The model under review builds one solid part; all positions refer to its coordinate system, in mm. A direction names the side the tool comes from. Round coordinates to 2 decimals unless told otherwise and drop trailing zeros. Write each loop counter-clockwise with the first axis right and the second up, starting at its lowest first coordinate (ties: lowest second). Pieces come first, ordered by that corner, then holes. Notation, with made-up numbers: (66, -7) - (105, -7) arc R19 cw to (105, 4) - close; hole circle Ø1 at (-2, 79.5). An arc over 180 degrees is marked (long way). Return JSON: item names as keys, results as strings.
from build123d import *
from build123d.topology import SkipClean

# Parameters (mm, degrees)
EXTRUDE_1_DEPTH     = 10
CUT_EXTRUDE_1_DEPTH = 5


with BuildPart() as part:
    # 草圖1 → 填料-伸長1 (new, symmetric)
    with BuildSketch(Plane(origin=(0, 0, 0), x_dir=(1, 0, 0), z_dir=(0, 1, 0))):
        with BuildLine():
            Line((95.00000000000004, 14.999999999999998), (-94.99999999999996, 15))
            ThreePointArc((-94.99999999999996, 14.999999999999998), (-84.39339828220174, 10.606601717798211), (-79.99999999999996, 0))
            ThreePointArc((-79.99999999999996, -3.67e-15), (-84.39339828220174, -10.606601717798204), (-94.99999999999994, -14.999999999999998))
            Line((-94.99999999999994, -14.999999999999961), (95.00000000000006, -14.999999999999998))
            ThreePointArc((95.00000000000004, -14.999999999999998), (80.00000000000004, 1.84e-15), (95.00000000000004, 14.999999999999998))
        make_face()
        with BuildLine():
            ThreePointArc((-79.99999999999996, 0), (-84.39339828220174, 10.606601717798211), (-94.99999999999996, 14.999999999999998))
            Line((-94.99999999999996, 15), (-94.99999999999996, 10.000000000000009))
            ThreePointArc((-95, 10.000000000000009), (-87.9289321881345, 7.071067811865497), (-84.99999999999994, 0))
            ThreePointArc((-84.99999999999994, -2.45e-15), (-87.9289321881345, -7.071067811865502), (-95, -10.000000000000009))
            Line((-94.99999999999994, -10.000000000000007), (-94.99999999999994, -14.999999999999961))
            ThreePointArc((-94.99999999999994, -14.999999999999998), (-84.39339828220174, -10.606601717798204), (-79.99999999999996, -3.67e-15))
        make_face()
        with BuildLine():
            Line((-94.99999999999996, 10.000000000000009), (-94.99999999999996, 15))
            ThreePointArc((-94.99999999999996, 14.999999999999998), (-109.99999999999996, -4.82e-15), (-94.99999999999994, -14.999999999999998))
            Line((-94.99999999999994, -14.999999999999961), (-94.99999999999994, -10.000000000000007))
            ThreePointArc((-95, -10.000000000000009), (-104.99999999999997, 1.22e-15), (-95, 10.000000000000009))
        make_face()
        with BuildLine():
            ThreePointArc((-79.99999999999996, 0), (-84.39339828220174, 10.606601717798211), (-94.99999999999996, 14.999999999999998))
            Line((-94.99999999999996, 15), (-94.99999999999996, 10.000000000000009))
            ThreePointArc((-95, 10.000000000000009), (-87.9289321881345, 7.071067811865497), (-84.99999999999994, 0))
            ThreePointArc((-84.99999999999994, -2.45e-15), (-87.9289321881345, -7.071067811865502), (-95, -10.000000000000009))
            Line((-94.99999999999994, -10.000000000000007), (-94.99999999999994, -14.999999999999961))
            ThreePointArc((-94.99999999999994, -14.999999999999998), (-84.39339828220174, -10.606601717798204), (-79.99999999999996, -3.67e-15))
        make_face()
        with BuildLine():
            Line((-94.99999999999996, 10.000000000000009), (-94.99999999999996, 15))
            ThreePointArc((-94.99999999999996, 14.999999999999998), (-109.99999999999996, -4.82e-15), (-94.99999999999994, -14.999999999999998))
            Line((-94.99999999999994, -14.999999999999961), (-94.99999999999994, -10.000000000000007))
            ThreePointArc((-95, -10.000000000000009), (-104.99999999999997, 1.22e-15), (-95, 10.000000000000009))
        make_face()
        with BuildLine():
            ThreePointArc((110.00000000000004, 0), (105.60660171779826, 10.606601717798211), (95.00000000000004, 14.999999999999998))
            Line((95.00000000000004, 14.999999999999998), (95.00000000000004, 10.000000000000009))
            ThreePointArc((95, 10.000000000000009), (102.0710678118655, 7.071067811865497), (105.00000000000006, 0))
            ThreePointArc((105.00000000000006, -2.45e-15), (102.0710678118655, -7.071067811865502), (95, -10.000000000000009))
            Line((95.00000000000004, -10.000000000000009), (95.00000000000004, -14.999999999999998))
            ThreePointArc((95.00000000000004, -14.999999999999998), (105.60660171779826, -10.606601717798213), (110.00000000000004, -3.67e-15))
        make_face()
        with BuildLine():
            Line((95.00000000000004, 10.000000000000009), (95.00000000000004, 14.999999999999998))
            ThreePointArc((95.00000000000004, 14.999999999999998), (80.00000000000004, 1.84e-15), (95.00000000000004, -14.999999999999998))
            Line((95.00000000000004, -14.999999999999998), (95.00000000000004, -10.000000000000009))
            ThreePointArc((95, -10.000000000000009), (85.00000000000003, 1.22e-15), (95, 10.000000000000009))
        make_face()
        with BuildLine():
            ThreePointArc((110.00000000000004, 0), (105.60660171779826, 10.606601717798211), (95.00000000000004, 14.999999999999998))
            Line((95.00000000000004, 14.999999999999998), (95.00000000000004, 10.000000000000009))
            ThreePointArc((95, 10.000000000000009), (102.0710678118655, 7.071067811865497), (105.00000000000006, 0))
            ThreePointArc((105.00000000000006, -2.45e-15), (102.0710678118655, -7.071067811865502), (95, -10.000000000000009))
            Line((95.00000000000004, -10.000000000000009), (95.00000000000004, -14.999999999999998))
            ThreePointArc((95.00000000000004, -14.999999999999998), (105.60660171779826, -10.606601717798213), (110.00000000000004, -3.67e-15))
        make_face()
        with BuildLine():
            Line((95.00000000000004, 10.000000000000009), (95.00000000000004, 14.999999999999998))
            ThreePointArc((95.00000000000004, 14.999999999999998), (80.00000000000004, 1.84e-15), (95.00000000000004, -14.999999999999998))
            Line((95.00000000000004, -14.999999999999998), (95.00000000000004, -10.000000000000009))
            ThreePointArc((95, -10.000000000000009), (85.00000000000003, 1.22e-15), (95, 10.000000000000009))
        make_face()
    extrude(amount=EXTRUDE_1_DEPTH, both=True)

    # 草圖2 → 除料-伸長1 (cut, symmetric)
    with SkipClean():  # the faces are left unmerged after this step: merging them gives an invalid solid
        with BuildSketch(Plane(origin=(0, 0, 0), x_dir=(1, 0, 0), z_dir=(0, 1, 0))):
            with BuildLine():
                Line((-44.99999999999994, 14.99999999999999), (-44.99999999999996, -14.999999999999977))
                Line((-44.99999999999996, -14.999999999999977), (-94.99999999999994, -14.99999999999998))
                ThreePointArc((-94.99999999999994, -14.99999999999998), (-109.99999999999994, -4.82e-15), (-94.99999999999996, 14.99999999999998))
                Line((-94.99999999999996, 14.99999999999998), (-44.99999999999994, 14.99999999999999))
            make_face()
        cut_extrude_1 = extrude(amount=CUT_EXTRUDE_1_DEPTH, both=True, mode=Mode.SUBTRACT)

    # 鏡射1: 除料-伸長1 across plane
    with SkipClean():  # the faces are left unmerged after this step: merging them gives an invalid solid
        add(cut_extrude_1.mirror(Plane(origin=(0, 0, 0), x_dir=(0, 0, 1), z_dir=(1, 0, 0))), mode=Mode.SUBTRACT)


solid = part.part
(1) For faces 1 (the flat face through (77, 5, 0)), 2 (the flat face through (-77, -5, 0)), 3 (the cylindrical face through (-85.24, 7.54, -2.17)), list the 3-axis set-ups (+Z, -Z, +X, -X, +Y, -Y) from which the entire face can be reached by the end or side of a thin tool; tool diameter is ignored.
Filled in:
{"face 1": "+Z, -Z, +X", "face 2": "+Z, -Z, -X", "face 3": "+Y, -Y"}
(2) Add section D-D (z = -12.5). Write out the cut boundary in (x, y), plus the area to 3 significant figures.
Filled in:
{"outline": "(-103.29, -10) - (103.29, -10) - (103.29, -5) - (45, -5) - (45, 5) - (103.29, 5) - (103.29, 10) - (-103.29, 10) - (-103.29, 5) - (-45, 5) - (-45, -5) - (-103.29, -5) - close", "area": "2,970 mm2"}
(3) Clearance check with flat-ended pins moving along their axes: pin 1 Ø4 at (y, z) = (-4, -5) entering from +X; pin 2 Ø3 at (y, z) = (-4.5, 6.5) entering from +X; pin 3 Ø1 at (y, z) = (3, 8.5) entering from -X; pin 4 Ø8 at (x, y) = (-48.5, -2) entering from -Z. State where each tip first meets the part, or that it passes through.
Filled in:
{"pin 1": "stops at x = 109.64", "pin 2": "stops at x = 109.11", "pin 3": "stops at x = -45", "pin 4": "stops at z = -15"}
(4) Add section A-A (x = -51). Write out the cut boundary in (y, z), plus the area to 3 significant figures.
Filled in:
{"outline": "(-10, -15) - (-5, -15) - (-5, 15) - (-10, 15) - close; (5, -15) - (10, -15) - (10, 15) - (5, 15) - close", "area": "300 mm2"}
(5) Wall thickness on line 1 (X direction, y = -8.65, z = 0); line 2 (Y direction, x = -64.5, z = -12.5); line 3 (X direction, y = 7.5, z = -4.5): over which ranges is each line inside the solid? List them lowest first.
Filled in:
{"line 1": "x = -110 to -105, -85 to 85, 105 to 110", "line 2": "y = -10 to -5, 5 to 10", "line 3": "x = -109.31 to -103.93, -86.07 to 86.07, 103.93 to 109.31"}
(6) Add section C-C (y = -0.5). Write out the cut boundary in (x, z), plus the area to 3 significant figures.
Filled in:
{"outline": "(-45, -15) - (45, -15) - (45, 15) - (-45, 15) - close", "area": "2,700 mm2"}
(7) Add section B-B (z = 0). Write out the cut boundary in (x, y), plus the area to 3 significant figures.
Filled in:
{"outline": "(-110, -10) - (-105, -10) - (-105, -5) - (-110, -5) - close; (-110, 5) - (-105, 5) - (-105, 10) - (-110, 10) - close; (-85, -10) - (85, -10) - (85, -5) - (45, -5) - (45, 5) - (85, 5) - (85, 10) - (-85, 10) - (-85, 5) - (-45, 5) - (-45, -5) - (-85, -5) - close; (105, -10) - (110, -10) - (110, -5) - (105, -5) - close; (105, 5) - (110, 5) - (110, 10) - (105, 10) - close", "area": "2,700 mm2"}
(8) Mouldability with a two-part tool opening along X and no side actions: class faces 4 (the cylindrical face through (104.915, -7.465, 1.302)), 5 (the flat face through (-1, 0, 15)), 6 (the cylindrical face through (104.915, 7.535, 1.302)), 7 (the cylindrical face through (-110, -7, 0)) as released by +X, released by -X, zero draft, split by the parting line, or undercut.
Filled in:
{"face 4": "undercut", "face 5": "zero draft", "face 6": "undercut", "face 7": "released by -X"}
